from build123d import *

# Parameters (mm, degrees)
SKETCH_R        = 13.5
PAD_DEPTH       = 17.5
PAD001_DEPTH    = 10
POCKET_DEPTH    = 12
POCKET001_DEPTH = 5


with BuildPart() as part:
    # Sketch → Pad (new body)
    with BuildSketch(Plane.XY):
        Circle(SKETCH_R)
    extrude(amount=PAD_DEPTH)

    # Sketch001 (on Face3 of Pad) → Pad001 (join)
    with BuildSketch(Plane.XY.offset(17.5)):
        Polygon((12, 0), (6, 10.392305), (-6, 10.392305), (-12, 0), (-6, -10.392305), (6, -10.392305), align=None)
    extrude(amount=PAD001_DEPTH)

    # Sketch002 (on Face10 of Pad001) → Pocket (cut)
    with BuildSketch(Plane.XY.offset(27.5)):
        Polygon((6.062178, 0), (3.031089, 5.25), (-3.031089, 5.25), (-6.062178, 0), (-3.031089, -5.25), (3.031089, -5.25), align=None)
    extrude(amount=-POCKET_DEPTH, mode=Mode.SUBTRACT)

    # Sketch003 (on Face2 of Pocket) → Pocket001 (cut)
    with BuildSketch(Plane(origin=(0, 0, 0), x_dir=(1, 0, 0), z_dir=(0, 0, -1))):
        with BuildLine():
            Line((-4.5, 12.727922), (-4.5, 5.5))
            Line((-4.5, 5.5), (4.5, 5.5))
            Line((4.5, 5.5), (4.5, 12.727922))
            ThreePointArc((4.5, 12.727922), (0, 13.5), (-4.5, 12.727922))
        make_face()
        with BuildLine():
            Line((-4.5, -5.5), (4.5, -5.5))
            Line((4.5, -5.5), (4.5, -12.727922))
            ThreePointArc((-4.5, -12.727922), (0, -13.5), (4.5, -12.727922))
            Line((-4.5, -12.727922), (-4.5, -5.5))
        make_face()
    extrude(amount=-POCKET001_DEPTH, mode=Mode.SUBTRACT)


solid = part.part
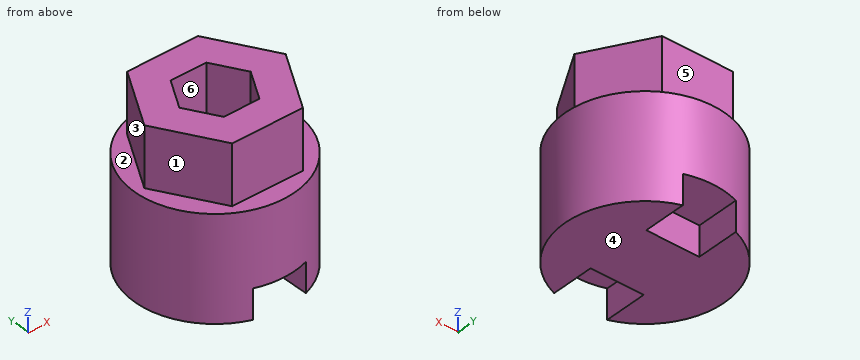
Can you work these out from the model? Positions are in its coordinate system, mm. Face numbers are marked on the shaded views. A direction names the side the tool comes from. Coordinates: 2 decimals unless noted, no trailing zeros. Loops run counter-clockwise (first coordinate to the right, second up) from the corner with the lowest first, then second, coordinate; pieces in that order, holes last. Notation, with made-up numbers: (29.25, 68) - (81.25, 68) arc R9 ccw to (81.25, 80) - close; hole circle Ø1 at (53.25, -14). An arc over 180 degrees is marked (long way). Answer as a JSON object with one key per item and string values. Group by question number.
Item 1: If I drill on L1, parallel to Z at x = -11, y = 3; L2, parallel to X at y = -8.5, z = 3; L3, parallel to X at y = -6.75, z = 3, over which ranges is the centre line in solid material (lowest first)? Write a range as from..to.
Item 2: For pin 1 (5.5 mm diameter, centred on y = 8.5, z = 3.5, fed in from -X); pin 2 (1 mm diameter, centred on y = -1, z = 21, fed in from +X); pin 3 (4 mm diameter, centred on x = 0.5, z = 2.5, fed in from -Y), each with a flat end and sliding along its axis, tell me the tip position at first contact or that it passes through.
Item 3: If we section it at A-A (z = 19.5): List the corners of the cut face in (x, y) for me.
Item 4: If we section it at D-D (y = 8.75): List the corners of the cut face in (x, z) for me, plus the area to 3 significant figures.
Item 5: If we section it at B-B (x = 0): List the corners of the cut face in (y, z) for me.
Item 6: If we section it at C-C (z = 3.25): List the corners of the cut face in (x, y) for me.
Item 7: On a 3-axis mill with a long thin cutter (end or side, diameter ignored), from which of +Z, -Z, +X, -X, +Y, -Y can I reach the whole of each face in a straight line? I mean the marked faces 1, 2 and 3. Say none if no direction works.
Item 8: If we mould it in two halves opening along Y, with no side actions, what happens to the marked faces 4, 5 and 6? For each: released by +Y, released by -Y, zero draft, split by the parting line, or undercut.
Returned:
{
 "1": {"L1": "z = 0..17.5", "L2": "x = -10.49..-4.5, 4.5..10.49", "L3": "x = -11.69..-4.5, 4.5..11.69"},
 "2": {"pin 1": "stops at x = -12.21", "pin 2": "stops at x = 11.71", "pin 3": "stops at y = -5.5"},
 "3": {"outline": "(-12, 0) - (-6, -10.39) - (6, -10.39) - (12, 0) - (6, 10.39) - (-6, 10.39) - close; hole (-6.06, 0) - (-3.03, -5.25) - (3.03, -5.25) - (6.06, 0) - (3.03, 5.25) - (-3.03, 5.25) - close"},
 "4": {"outline": "(-10.28, 0) - (-4.5, 0) - (-4.5, 5) - (4.5, 5) - (4.5, 0) - (10.28, 0) - (10.28, 17.5) - (6.95, 17.5) - (6.95, 27.5) - (-6.95, 27.5) - (-6.95, 17.5) - (-10.28, 17.5) - close", "area": "454 mm²"},
 "5": {"outline": "(-13.5, 5) - (-5.5, 5) - (-5.5, 0) - (5.5, 0) - (5.5, 5) - (13.5, 5) - (13.5, 17.5) - (10.39, 17.5) - (10.39, 27.5) - (5.25, 27.5) - (5.25, 15.5) - (-5.25, 15.5) - (-5.25, 27.5) - (-10.39, 27.5) - (-10.39, 17.5) - (-13.5, 17.5) - close"},
 "6": {"outline": "(-4.5, -12.73) - (-4.5, -5.5) - (4.5, -5.5) - (4.5, -12.73) arc R13.5 ccw to (4.5, 12.73) - (4.5, 5.5) - (-4.5, 5.5) - (-4.5, 12.73) arc R13.5 ccw to start"},
 "7": {"face 1": "+Z, -X, -Y", "face 2": "+Z", "face 3": "+Z, -X, +Y"},
 "8": {"face 4": "zero draft", "face 5": "released by +Y", "face 6": "undercut"}
}
